Read the model definition and answer for the solid it produces. Units are mm, in the model's axes. Face numbers are marked on the shaded views. A direction names the side the tool comes from. Coordinates: 2 decimals unless noted, no trailing zeros. Loops run counter-clockwise (first coordinate to the right, second up) from the corner with the lowest first, then second, coordinate; pieces in that order, holes last.
from build123d import *

# Parameters (mm, degrees)
SKETCH1_W           = 50
SKETCH1_H           = 25
SKETCH1_R           = 1.6
BOSS_EXTRUDE1_DEPTH = 1.5875
SKETCH2_W           = 50
SKETCH2_H           = 12.870978344
BOSS_EXTRUDE2_DEPTH = 1.5875
SKETCH3_R           = 0.46355
CUT_EXTRUDE1_DEPTH  = 1.5875


with BuildPart() as part:
    # Sketch1 → Boss-Extrude1 (new body)
    with BuildSketch(Plane.XY):
        Rectangle(SKETCH1_W, SKETCH1_H)
        with Locations((-18.5, 0)):
            Circle(SKETCH1_R, mode=Mode.SUBTRACT)
        with Locations((18.5, 0)):
            Circle(SKETCH1_R, mode=Mode.SUBTRACT)
    extrude(amount=BOSS_EXTRUDE1_DEPTH)

    # Sketch2 → Boss-Extrude2 (add)
    with BuildSketch(Plane(origin=(0, 12.5, 0), x_dir=(1, 0, 0), z_dir=(0, 1, 0))):
        with Locations((0, 6.435489172)):
            Rectangle(SKETCH2_W, SKETCH2_H)
    extrude(amount=-BOSS_EXTRUDE2_DEPTH)

    # Sketch3 → Cut-Extrude1 (cut)
    with BuildSketch(Plane(origin=(0, 12.5, 0), x_dir=(1, 0, 0), z_dir=(0, 1, 0))):
        with Locations(Location((-14.1859, 5.641739172, 0), (0, 0, 270))):
            Circle(SKETCH3_R)
        with Locations(Location((14.1859, 5.641739172, 0), (0, 0, 270))):
            Circle(SKETCH3_R)
    extrude(amount=-CUT_EXTRUDE1_DEPTH, mode=Mode.SUBTRACT)


solid = part.part
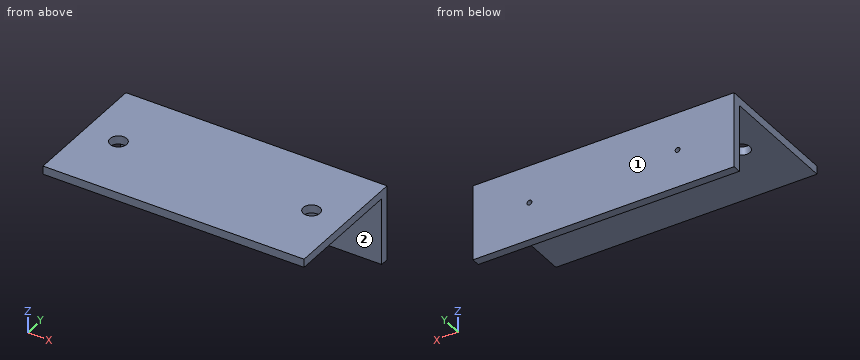
Item 1: Which of the six approach directions +Z, -Z, +X, -X, +Y, -Y give full straight-line access (tool end or side, diameter ignored) to the marked faces 1 and 2?
Numbers:
face 1: +Z, -Z, +X, -X, +Y
face 2: -Z, +X, -X, -Y
Item 2: A cutting plane is placed at D-D on y = 3.75. Determine the outline of the cut face in (x, z), then the cut area to 3 significant figures.
Numbers:
outline: (-25, 0) - (25, 0) - (25, 1.59) - (-25, 1.59) - close
area: 79.4 mm2
Item 3: Given pin 1 (1.5 mm diameter, centred on x = 13.5, y = 5, fed in from -Z); pin 2 (6.5 mm diameter, centred on x = -5, z = -6.5, fed in from -Y), each flat-ended and moving along its own axis, determine where each tip first touches the part or whether it passes through.
Numbers:
pin 1: stops at z = 0
pin 2: stops at y = 10.91
Item 4: A cutting plane is placed at B-B on x = -18.5. Determine the outline of the cut face in (y, z).
Numbers:
outline: (-12.5, 0) - (-1.6, 0) - (-1.6, 1.59) - (-12.5, 1.59) - close; (1.6, 0) - (10.91, 0) - (10.91, -12.87) - (12.5, -12.87) - (12.5, 1.59) - (1.6, 1.59) - close
Item 5: A cutting plane is placed at A-A on y = 0. Determine the outline of the cut face in (x, z).
Numbers:
outline: (-25, 0) - (-20.1, 0) - (-20.1, 1.59) - (-25, 1.59) - close; (-16.9, 0) - (16.9, 0) - (16.9, 1.59) - (-16.9, 1.59) - close; (20.1, 0) - (25, 0) - (25, 1.59) - (20.1, 1.59) - close
Item 6: Find the intervals of material crossed by line 1 along Y through (x, z) = (18.5, 0.8); line 2 along Y through (x, z) = (-1, -0.25); line 3 along Z through (x, y) = (9.5, 9), in increasing order.
Numbers:
line 1: y = -12.5 to -1.6, 1.6 to 12.5
line 2: y = 10.91 to 12.5
line 3: z = 0 to 1.59
Item 7: A cutting plane is placed at C-C on z = -7.5. Determine the outline of the cut face in (x, y), then the cut area to 3 significant figures.
Numbers:
outline: (-25, 10.91) - (25, 10.91) - (25, 12.5) - (-25, 12.5) - close
area: 79.4 mm2
